Autodesk Inventor part; units mm, degrees
ref_plane "YZ Plane" through (0, 0, 0) normal (1, 0, 0) x (0, 1, 0)
ref_plane "XZ Plane" through (0, 0, 0) normal (0, 1, 0) x (-1, 0, 0)
ref_plane "XY Plane" through (0, 0, 0) normal (0, 0, 1) x (1, 0, 0)
sketch "Sketch1" plane through (0, 0, 0) normal (0, 1, 0) x (-1, 0, 0)
  line L0 (100, 65) -> (-100, 65)
  line L1 (-100, 65) -> (-100, -65)
  line L2 (-100, -65) -> (100, -65)
  line L3 (100, -65) -> (100, 65)
  line L4 (100, 65) -> (-100, -65) construction
  line L5 (-100, 65) -> (100, -65) construction
  circle A0 centre (100, 65) radius 6
  circle A1 centre (-100, -65) radius 6
  point P0 (0, 0)
  point P1 (94, 65)
  point P2 (100, 59)
  point P3 (-100, -59)
  point P4 (-94, -65)
  dimension "d0" = 200
  dimension "d1" = 130
  dimension "d4" = 12
extrude "Extrusion1" add sketch "Sketch1" along normal blind 5
fillet "Fillet1" radius 2 2 edges at (100, 2.5, 65) (-100, 2.5, -65)
sketch "Sketch2" plane through (0, 5, 0) normal (0, 1, 0) x (1, 0, 0)
  arc A0 (-98, 65) -> (-100, 63) centre (-98, 63) ccw
  line L0 (-100, 63) -> (-100, -59)
  arc A1 (-100, -59) -> (-94, -65) centre (-100, -65) ccw
  line L1 (-94, -65) -> (98, -65)
  arc A2 (98, -65) -> (100, -63) centre (98, -63) ccw
  line L2 (100, -63) -> (100, 59)
  arc A3 (100, 59) -> (94, 65) centre (100, 65) ccw
  line L3 (94, 65) -> (-98, 65)
  point P0 (0, 0)
hole "Hole1" at (100, 5, -65) at (-100, 5, 65) direction (0, -1, 0) diameter 3.2 end through all
sketch "Sketch3" plane through (0, 5, 0) normal (0, 1, 0) x (1, 0, 0)
  circle A0 centre (0, 0) radius 40
  dimension "d13" = 80
extrude "Extrusion2" cut sketch "Sketch3" against normal through all
sketch "Sketch4" plane through (0, 5, 0) normal (0, 1, 0) x (1, 0, 0)
  line L0 (-35.75, -35.75) -> (35.75, -35.75) construction
  line L1 (35.75, -35.75) -> (35.75, 35.75) construction
  line L2 (35.75, 35.75) -> (-35.75, 35.75) construction
  line L3 (-35.75, 35.75) -> (-35.75, -35.75) construction
  line L4 (-35.75, -35.75) -> (35.75, 35.75) construction
  line L5 (35.75, -35.75) -> (-35.75, 35.75) construction
  point P0 (0, 0)
  dimension "d16" = 71.5
hole "Hole2" at (-35.75, 5, -35.75) at (-35.75, 5, 35.75) at (35.75, 5, 35.75) at (35.75, 5, -35.75) direction (0, -1, 0) diameter 3.7 end through all
sketch "Sketch5" plane through (0, 5, 0) normal (0, 1, 0) x (1, 0, 0)
  line L0 (-52.5, 7) -> (-47.5, 7)
  line L1 (-47.5, 7) -> (-47.5, -3)
  line L2 (-47.5, -3) -> (-52.5, -3)
  line L3 (-52.5, -3) -> (-52.5, 7)
  line L4 (-52.5, 7) -> (-47.5, -3) construction
  line L5 (-47.5, 7) -> (-52.5, -3) construction
  line L6 (-100, 63) -> (-100, -59)
  point P0 (0, 0)
  point P1 (-50, 2)
  point P2 (-100, 2)
  point P3 (-100, 2)
  dimension "d24" = 50
  dimension "d25" = 5
  dimension "d26" = 10
extrude "Extrusion3" cut sketch "Sketch5" against normal through all
properties part number "LED Power Box (12V) Cover" material "ABS Plastic"
Work out the finished part from the listing and answer in its coordinate system (mm). A direction names the side the tool comes from. Give positions to 0.01 mm unless a question says otherwise; leave off trailing zeros. Order: outer loops, then holes, each group sorted by start corner. A loop starts at its lowest first (then second) coordinate and runs counter-clockwise, first axis right, second up. Notation, with made-up numbers: M -21,45.25 L 11,45.25 A19 ccw 11,51.25 Z; hole C 37,8 d9. An arc over 180 degrees is marked long. Return JSON: item names as keys, results as strings.
1) Straight lines are drawn through the part: line 1 along Z through (x, y) = (-35.75, 1.55); line 2 along X through (y, z) = (4.65, -34.5); line 3 along Z through (x, y) = (-50.5, 1.45). For each, find the intervals that lie inside material, in ascending order. Write a range as [from, to].
Resolved:
{"line 1": "[-65, -37.6], [-33.9, -17.94], [17.94, 33.9], [37.6, 65]", "line 2": "[-100, -37.11], [-34.39, -20.24], [20.24, 34.39], [37.11, 100]", "line 3": "[-65, -7], [3, 65]"}
2) Section B-B, the plane x = 0 is taken. Write down the section's boundary in (y, z).
Resolved:
{"outline": "M 0,-65 L 5,-65 L 5,-40 L 0,-40 Z; M 0,40 L 5,40 L 5,65 L 0,65 Z"}
3) Section D-D, the plane z = 54.5 is taken. Write down the section's boundary in (x, y).
Resolved:
{"outline": "M -100,0 L 100,0 L 100,5 L -100,5 Z"}
4) Each of these flat-tipped pins is pushed along its axis until it touches: pin 1 (1.5 mm diameter, centred on x = -49, y = 2, fed in from +Z); pin 2 (2.5 mm diameter, centred on y = 2, z = 0, fed in from -X); pin 3 (2.5 mm diameter, centred on y = 3, z = 0.5, fed in from +X). Where does it stop, or does it pass through?
Resolved:
{"pin 1": "z = 65", "pin 2": "x = -100", "pin 3": "x = 100"}
5) For a pull along X with two mould halves and no side action, classify faces 6 (the flat face through (-50, 3, -7)), 7 (the flat face through (-1, 2, -65)), 8 (the cylindrical face through (104.1, 2.46, -69.38)), 9 (the flat face through (-52.5, 3, -2)) as +X half, -X half, draft (parallel to the pull), parting line (faces both ways), or undercut.
Resolved:
{"face 6": "undercut", "face 7": "draft", "face 8": "parting line", "face 9": "undercut"}
6) Section C-C, the plane y = 2.5 is taken. Give the number of separate pieces and of enclosed holes in the cut face, plus the area to 3 significant figures.
Resolved:
{"separate pieces": "1", "enclosed holes": "8", "area": "21,000 mm^2"}
7) Section A-A, the plane z = 0 is taken. Write down the section's boundary in (x, y), plus the area to 3 significant figures.
Resolved:
{"outline": "M -100,0 L -52.5,0 L -52.5,5 L -100,5 Z; M -47.5,0 L -40,0 L -40,5 L -47.5,5 Z; M 40,0 L 100,0 L 100,5 L 40,5 Z", "area": "575 mm^2"}
8) A tool of negligible diameter and unlimited length cuts with its end or side. For faces 1 (the flat face through (1, 2, 65)), 2 (the flat face through (25, 0, 33)), 3 (the flat face through (25, 5, 33)), 4 (the flat face through (-100, 2, -3)), 5 (the flat face through (-50, 3, 3)), from which of +Z, -Z, +X, -X, +Y, -Y can it reach the whole face along a straight path? Write none if from no direction.
Resolved:
{"face 1": "+Z, +X, +Y, -Y", "face 2": "+Z, -Z, +X, -X, -Y", "face 3": "+Z, -Z, +X, -X, +Y", "face 4": "-Z, -X, +Y, -Y", "face 5": "+Y, -Y"}
